Verification items for the finished model (mm, model axes). Coordinates: 2 decimals unless noted, no trailing zeros. Order: outer loops, then holes, each group sorted by start corner. A loop starts at its lowest first (then second) coordinate and runs counter-clockwise, first axis right, second up. Notation, with made-up numbers: (54, -37) -> (70, -37) arc R30 cw to (70, -12) -> close; hole circle Ø2 at (11.5, -10). An arc over 180 degrees is marked (long way). Write item = value, one per line. Start each with the question number.
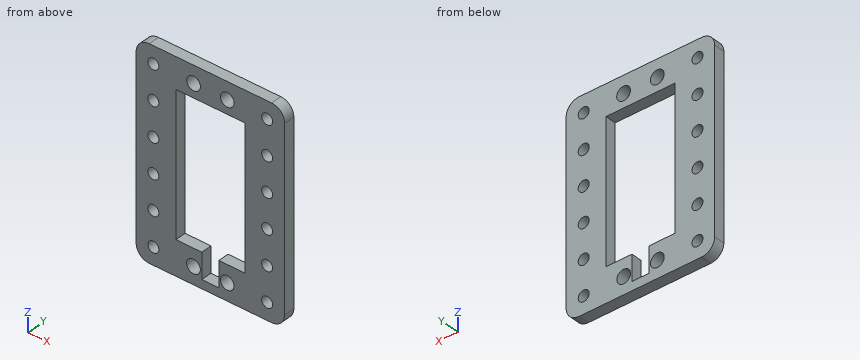
from build123d import *

# Parameters (mm, degrees)
F0_R     = 1.6
F0_R_2   = 2
F1_DEPTH = 3.175


# Not quite as in the source:
# - a length typed as a fraction of an inch, garbled in the dataset ("3 / 203.2 mm" for 3/8 in), is restored


with BuildPart() as f1:
    # F0 (on Front) → F1 (new body)
    with BuildSketch(Plane.XZ):
        with BuildLine():
            Line((27.8025, 8.975), (-7.7525, 8.975))
            ThreePointArc((-7.7525, 8.975), (-10.4465768363, 7.8590768363), (-11.5625, 5.165))
            Line((-11.5625, 5.165), (-11.5625, -47.215))
            ThreePointArc((-11.5625, -47.215), (-10.4465768363, -49.9090768363), (-7.7525, -51.025))
            Line((-7.7525, -51.025), (27.8025, -51.025))
            ThreePointArc((27.8025, -51.025), (30.4965768363, -49.9090768363), (31.6125, -47.215))
            Line((31.6125, -47.215), (31.6125, 5.165))
            ThreePointArc((31.6125, 5.165), (30.4965768363, 7.8590768363), (27.8025, 8.975))
        make_face()
        with Locations((-6.5625, -46.025)):
            Circle(F0_R, mode=Mode.SUBTRACT)
        with Locations((5.1, -46.025)):
            Circle(F0_R_2, mode=Mode.SUBTRACT)
        with Locations((-6.5625, -36.025)):
            Circle(F0_R, mode=Mode.SUBTRACT)
        with Locations((-6.5625, -26.025)):
            Circle(F0_R, mode=Mode.SUBTRACT)
        Polygon((0, -41), (0, 0), (20.025, 0), (20.025, -41.025), (12.4728614733, -41.025), (12.4728614733, -48.485), (7.5228614733, -48.485), (7.5228614733, -41.025), align=None, mode=Mode.SUBTRACT)
        with Locations((14.9, -46.025)):
            Circle(F0_R_2, mode=Mode.SUBTRACT)
        with Locations((26.5125, -46.025)):
            Circle(F0_R, mode=Mode.SUBTRACT)
        with Locations((26.5125, -36.025)):
            Circle(F0_R, mode=Mode.SUBTRACT)
        with Locations((26.5125, -26.025)):
            Circle(F0_R, mode=Mode.SUBTRACT)
        with Locations((-6.5625, -16.025)):
            Circle(F0_R, mode=Mode.SUBTRACT)
        with Locations((-6.5625, -6.025)):
            Circle(F0_R, mode=Mode.SUBTRACT)
        with Locations((-6.5625, 3.975)):
            Circle(F0_R, mode=Mode.SUBTRACT)
        with Locations((5.125, 3.975)):
            Circle(F0_R_2, mode=Mode.SUBTRACT)
        with Locations((26.5125, -16.025)):
            Circle(F0_R, mode=Mode.SUBTRACT)
        with Locations((14.925, 3.975)):
            Circle(F0_R_2, mode=Mode.SUBTRACT)
        with Locations((26.5125, -6.025)):
            Circle(F0_R, mode=Mode.SUBTRACT)
        with Locations((26.5125, 3.975)):
            Circle(F0_R, mode=Mode.SUBTRACT)
    extrude(amount=F1_DEPTH)


solid = f1.part
Item 1: Section check D-D (x = 2). Record the boundary of the cut face in (y, z) (3 decimals), then the cut area to 3 significant figures.
Item 2: Thickness scan on line 1 (X direction, y = -2.7, z = -16) (1 decimal); line 2 (X direction, y = -1.55, z = -9.5) (1 decimal); line 3 (Z direction, x = 14, y = -0.4) (3 decimals). Record the ranges inside material, lowest first.
Item 3: Section check C-C (y = -2). State how many separate pieces and enclosed holes the cut face has, then the cut area to 3 significant figures.
Item 4: Section check A-A (x = 10). Record the boundary of the cut face in (y, z) (3 decimals), then the cut area to 3 significant figures.
Item 5: Section check B-B (x = 14.9). Record the boundary of the cut face in (y, z) (3 decimals), then the cut area to 3 significant figures.
Filled sheet:
q1.outline = (-3.175, -51.025) -> (0, -51.025) -> (0, -41.007) -> (-3.175, -41.007) -> close; (-3.175, 0) -> (0, 0) -> (0, 8.975) -> (-3.175, 8.975) -> close
q1.area = 60.3 mm^2
q2.line_1 = -11.6 to -8.2, -5 to 0, 20 to 24.9, 28.1 to 31.6
q2.line_2 = -11.6 to 0, 20 to 31.6
q2.line_3 = -51.025 to -47.811, -44.239 to -41.025, 0 to 2.202, 5.748 to 8.975
q3.separate_pieces = 1
q3.enclosed_holes = 17
q3.area = 1,570 mm^2
q4.outline = (-3.175, -51.025) -> (0, -51.025) -> (0, -48.485) -> (-3.175, -48.485) -> close; (-3.175, 0) -> (0, 0) -> (0, 8.975) -> (-3.175, 8.975) -> close
q4.area = 36.6 mm^2
q5.outline = (-3.175, -51.025) -> (0, -51.025) -> (0, -48.025) -> (-3.175, -48.025) -> close; (-3.175, -44.025) -> (0, -44.025) -> (0, -41.025) -> (-3.175, -41.025) -> close; (-3.175, 0) -> (0, 0) -> (0, 1.975) -> (-3.175, 1.975) -> close; (-3.175, 5.975) -> (0, 5.975) -> (0, 8.975) -> (-3.175, 8.975) -> close
q5.area = 34.8 mm^2
